from build123d import *

# Parameters (mm, degrees)
BOSS_EXTRUDE1_DEPTH      = 9.525
BOSS_EXTRUDE1_DEPTH_BACK = 66.675
SKETCH1_W                = 25.4
SKETCH1_H                = 3.175
SKETCH2_W                = 25.4
SKETCH2_H                = 5.678954819
SKETCH2_R                = 2.38125
CUT_EXTRUDE1_DEPTH       = 204.193280927


with BuildPart() as part:
    # Sketch1 → Boss-Extrude1 (new, two sides: drawn at the far end of the back side and taken through both)
    with BuildSketch(Plane.XY.offset(-BOSS_EXTRUDE1_DEPTH_BACK)):
        with Locations((179.216318128, 372.614308443)):
            Rectangle(SKETCH1_W, SKETCH1_H)
    extrude(amount=BOSS_EXTRUDE1_DEPTH + BOSS_EXTRUDE1_DEPTH_BACK)

    # Sketch2 → Cut-Extrude1 (cut, through all)
    with BuildSketch(Plane(origin=(0, 374.201808443, 0), x_dir=(1, 0, 0), z_dir=(0, 1, 0))):
        with BuildLine():
            Line((166.516318128, 57.15), (166.516318128, 47.625))
            Line((166.516318128, 47.625), (169.691318128, 47.625))
            Line((169.691318128, 47.625), (169.691318128, 53.975))
            Line((169.691318128, 53.975), (172.866318128, 53.975))
            Line((172.866318128, 53.975), (172.866318128, 65.0875))
            ThreePointArc((172.866318128, 65.0875), (173.331286113, 66.210032015), (174.453818128, 66.675))
            Line((174.453818128, 66.675), (166.516318128, 66.675))
            Line((166.516318128, 66.675), (166.516318128, 57.15))
        make_face()
        with Locations((179.216318128, 69.51447741)):
            Rectangle(SKETCH2_W, SKETCH2_H)
        with BuildLine():
            Line((188.741318128, 47.625), (191.916318128, 47.625))
            Line((191.916318128, 47.625), (191.916318128, 53.975))
            Line((191.916318128, 53.975), (191.916318128, 66.675))
            Line((191.916318128, 66.675), (183.978818128, 66.675))
            ThreePointArc((183.978818128, 66.675), (185.101350143, 66.210032015), (185.566318128, 65.0875))
            Line((185.566318128, 65.0875), (185.566318128, 53.975))
            Line((185.566318128, 53.975), (188.741318128, 53.975))
            Line((188.741318128, 53.975), (188.741318128, 47.625))
        make_face()
        with Locations(Location((179.216318128, 62.70625, 0), (0, 0, 270))):
            Circle(SKETCH2_R)
        with BuildLine():
            Line((169.691318128, 9.525), (166.516318128, 9.525))
            Line((166.516318128, 9.525), (166.516318128, 0))
            Line((166.516318128, 0), (166.516318128, -9.525))
            Line((166.516318128, -9.525), (174.453818128, -9.525))
            ThreePointArc((174.453818128, -9.525), (173.331286113, -9.060032015), (172.866318128, -7.9375))
            Line((172.866318128, -7.9375), (172.866318128, 3.175))
            Line((172.866318128, 3.175), (169.691318128, 3.175))
            Line((169.691318128, 3.175), (169.691318128, 9.525))
        make_face()
        with Locations((179.216318128, -12.36447741)):
            Rectangle(SKETCH2_W, SKETCH2_H)
        with BuildLine():
            Line((191.916318128, 3.175), (191.916318128, 9.525))
            Line((191.916318128, 9.525), (188.741318128, 9.525))
            Line((188.741318128, 9.525), (188.741318128, 3.175))
            Line((188.741318128, 3.175), (185.566318128, 3.175))
            Line((185.566318128, 3.175), (185.566318128, -7.9375))
            ThreePointArc((185.566318128, -7.9375), (185.101350143, -9.060032015), (183.978818128, -9.525))
            Line((183.978818128, -9.525), (191.916318128, -9.525))
            Line((191.916318128, -9.525), (191.916318128, 3.175))
        make_face()
        with Locations(Location((179.216318128, -5.55625, 0), (0, 0, 90))):
            Circle(SKETCH2_R)
    extrude(amount=-CUT_EXTRUDE1_DEPTH, mode=Mode.SUBTRACT)


solid = part.part
Design review of the part built by this model. Coordinates are the model's own, in mm. A direction names the side the tool comes from. Give positions to 0.01 mm unless a question says otherwise; leave off trailing zeros. Loops run counter-clockwise (first coordinate to the right, second up) from the corner with the lowest first, then second, coordinate; pieces in that order, holes last. Notation, with made-up numbers: (64.5, 67) - (93.5, 67) arc R18 cw to (93.5, 86) - close; hole circle Ø3 at (45.25, 20.5). An arc over 180 degrees is marked (long way). Use CSV: the item, a comma, the result in double quotes. Start each with the question number.
1. Insertion check: P1, Ø1, axis at x = 168.5, y = 373, coming from the +Z side (3 decimals); P2, Ø1, axis at y = 372, z = -60, coming from the -X side; P3, Ø1, axis at x = 190.5, y = 373, coming from the -Z side (3 decimals). Each pin has a flat end and moves straight along its axis. Give the tip position at first contact, or say it passes through.
2. Wall thickness on L1, parallel to Z at x = 178, y = 373.5 (3 decimals); L2, parallel to Z at x = 170.75, y = 371.35 (3 decimals); L3, parallel to X at y = 372, z = -59: over which ranges is each line inside the solid? List them lowest first.
3. Add section B-B (y = 373.1). State the section outline as (x, z) points (1 decimal).
4. Draft analysis for pull direction X (two halves, no side actions). For faces 1 (the cylindrical face through (173.32, 372.64, -66.2)), 2 (the cylindrical face through (181.54, 372.64, 6.07)), 3 (the flat face through (179, 373, 9.525)), 4 (the cylindrical face through (185.11, 372.64, 9.05)), state which applies: released by +X, released by -X, zero draft, split by the parting line, or undercut.
5. Add section A-A (x = 180.5). State the section outline as (y, z) points (3 decimals), plus the area to 3 significant figures.
6. Add section D-D (x = 190). State the section outline as (y, z) points (3 decimals), plus the area to 3 significant figures.
7. Machinability: for faces 5 (the flat face through (190, 373, -47.625)), 6 (the flat face through (168, 373, -9.525)), 7 (the flat face through (179, 374.202, -29)), 8 (the flat face through (187, 373, -3.175)), 9 (the flat face through (172.866, 373, -59)), which of the approach directions +Z, -Z, +X, -X, +Y, -Y give a long, thin tool a straight path to every point of the face, cutting with its end or side? Answer none if there is none.
8. Add section C-C (z = -7.5). State the section outline as (x, y) points, plus the area to 3 significant figures.
Results found:
1,P1,"stops at z = -9.525"
1,P2,"stops at x = 172.87"
1,P3,"stops at z = -47.625"
2,L1,"z = -66.675 to -64.753, -60.659 to 3.509, 7.603 to 9.525"
2,L2,"z = -53.975 to -3.175"
2,L3,"x = 172.87 to 185.57"
3,outline,"(166.5, -47.6) - (169.7, -47.6) - (169.7, -54) - (172.9, -54) - (172.9, -65.1) arc R1.6 ccw to (174.5, -66.7) - (184, -66.7) arc R1.6 ccw to (185.6, -65.1) - (185.6, -54) - (188.7, -54) - (188.7, -47.6) - (191.9, -47.6) - (191.9, -9.5) - (188.7, -9.5) - (188.7, -3.2) - (185.6, -3.2) - (185.6, 7.9) arc R1.6 ccw to (184, 9.5) - (174.5, 9.5) arc R1.6 ccw to (172.9, 7.9) - (172.9, -3.2) - (169.7, -3.2) - (169.7, -9.5) - (166.5, -9.5) - close; hole circle Ø4.8 at (179.2, -62.7); hole circle Ø4.8 at (179.2, 5.6)"
4,face 1,"released by -X"
4,face 2,"undercut"
4,face 3,"zero draft"
4,face 4,"released by +X"
5,outline,"(371.027, -66.675) - (374.202, -66.675) - (374.202, -64.712) - (371.027, -64.712) - close; (371.027, -60.701) - (374.202, -60.701) - (374.202, 3.551) - (371.027, 3.551) - close; (371.027, 7.562) - (374.202, 7.562) - (374.202, 9.525) - (371.027, 9.525) - close"
5,area,"216 mm²"
6,outline,"(371.027, -47.625) - (374.202, -47.625) - (374.202, -9.525) - (371.027, -9.525) - close"
6,area,"121 mm²"
7,face 5,"-Z, +X, +Y, -Y"
7,face 6,"+Z, -X, +Y, -Y"
7,face 7,"+Z, -Z, +X, -X, +Y"
7,face 8,"+Z, +X, +Y, -Y"
7,face 9,"-Z, -X, +Y, -Y"
8,outline,"(169.69, 371.03) - (188.74, 371.03) - (188.74, 374.2) - (169.69, 374.2) - close"
8,area,"60.5 mm²"
